from build123d import *

# Parameters (mm, degrees)
SKETCH1_R           = 1.5
BOSS_EXTRUDE3_DEPTH = 15
SKETCH3_R           = 1.5
CUT_EXTRUDE1_DEPTH  = 7.5
SKETCH5_W           = 13
SKETCH5_H           = 24
CUT_EXTRUDE2_DEPTH  = 10
SKETCH6_R           = 1
CUT_EXTRUDE3_DEPTH  = 10
SKETCH8_R           = 5.15
CUT_EXTRUDE4_DEPTH  = 15
SKETCH9_W           = 3
SKETCH9_H           = 13
CUT_EXTRUDE5_DEPTH  = 16
FILLET2_R           = 2
SKETCH10_W          = 6
SKETCH10_H          = 1.8
CUT_EXTRUDE6_DEPTH  = 16
SKETCH11_R          = 0.75
CUT_EXTRUDE7_DEPTH  = 10
SKETCH13_R          = 1.5
CUT_EXTRUDE8_DEPTH  = 16
SKETCH14_R          = 3
CUT_EXTRUDE9_DEPTH  = 5
SKETCH15_W          = 9
SKETCH15_H          = 15
SKETCH15_R          = 1.15
BOSS_EXTRUDE4_DEPTH = 2
SKETCH16_W          = 31.135337716
SKETCH16_H          = 16.721473769
CUT_EXTRUDE10_DEPTH = 16
CUT_EXTRUDE11_DEPTH = 20


with BuildPart() as part:
    # Sketch1 → Boss-Extrude3 (new body)
    with BuildSketch(Plane(origin=(0, 0, 0), x_dir=(1, 0, 0), z_dir=(0, 1, 0))):
        with BuildLine():
            Line((17, 40), (17, -19))
            Line((17, -19), (-17, -19))
            Line((-17, -19), (-17, 40))
            ThreePointArc((-17, 40), (-14.071067812, 47.071067812), (-7, 50))
            Line((-7, 50), (7, 50))
            ThreePointArc((7, 50), (14.071067812, 47.071067812), (17, 40))
        make_face()
        with Locations((-9, 0)):
            Circle(SKETCH1_R, mode=Mode.SUBTRACT)
        with Locations((9, 0)):
            Circle(SKETCH1_R, mode=Mode.SUBTRACT)
    extrude(amount=BOSS_EXTRUDE3_DEPTH)

    # Sketch3 → Cut-Extrude1 (cut)
    with BuildSketch(Plane(origin=(0, 15, 0), x_dir=(1, 0, 0), z_dir=(0, 1, 0))):
        with Locations((-11, 43)):
            Circle(SKETCH3_R)
        with Locations((11, 43)):
            Circle(SKETCH3_R)
        with BuildLine():
            Line((6, 48), (-6, 48))
            Line((-6, 48), (-6, 43))
            ThreePointArc((-6, 43), (-7.171572875, 40.171572875), (-10, 39))
            Line((-10, 39), (-15, 39))
            Line((-15, 39), (-15, 6))
            Line((-15, 6), (15, 6))
            Line((15, 6), (15, 39))
            Line((15, 39), (10, 39))
            ThreePointArc((10, 39), (7.171572875, 40.171572875), (6, 43))
            Line((6, 43), (6, 48))
        make_face()
    extrude(amount=-CUT_EXTRUDE1_DEPTH, mode=Mode.SUBTRACT)

    # Sketch5 → Cut-Extrude2 (cut)
    with BuildSketch(Plane(origin=(0, 7.5, 0), x_dir=(1, 0, 0), z_dir=(0, 1, 0))):
        with Locations((0, 27)):
            Rectangle(SKETCH5_W, SKETCH5_H)
    extrude(amount=-CUT_EXTRUDE2_DEPTH, mode=Mode.SUBTRACT)

    # Sketch6 → Cut-Extrude3 (cut)
    with BuildSketch(Plane(origin=(0, 7.5, 0), x_dir=(1, 0, 0), z_dir=(0, 1, 0))):
        with Locations((0, 41.1)):
            Circle(SKETCH6_R)
        with Locations((0, 12.9)):
            Circle(SKETCH6_R)
    extrude(amount=-CUT_EXTRUDE3_DEPTH, mode=Mode.SUBTRACT)

    # Sketch8 → Cut-Extrude4 (cut)
    with BuildSketch(Plane(origin=(0, 15, 0), x_dir=(1, 0, 0), z_dir=(0, 1, 0))):
        with Locations((-6, -12)):
            Circle(SKETCH8_R)
        with Locations((6, -12)):
            Circle(SKETCH8_R)
    extrude(amount=-CUT_EXTRUDE4_DEPTH, mode=Mode.SUBTRACT)

    # Sketch9 → Cut-Extrude5 (cut, through all)
    with BuildSketch(Plane(origin=(0, 15, 0), x_dir=(1, 0, 0), z_dir=(0, 1, 0))):
        with Locations((15.5, -12.5)):
            Rectangle(SKETCH9_W, SKETCH9_H)
        with Locations((-15.5, -12.5)):
            Rectangle(SKETCH9_W, SKETCH9_H)
    extrude(amount=-CUT_EXTRUDE5_DEPTH, mode=Mode.SUBTRACT)

    # Fillet2
    fillet2_edges = [part.edges().sort_by_distance(p)[0] for p in [
        (14, 7.5, 19),
        (-14, 7.5, 19),
    ]]
    fillet(fillet2_edges, radius=FILLET2_R)

    # Sketch10 → Cut-Extrude6 (cut, through all)
    with BuildSketch(Plane(origin=(0, 15, 0), x_dir=(1, 0, 0), z_dir=(0, 1, 0))):
        with Locations((0, -18.1)):
            Rectangle(SKETCH10_W, SKETCH10_H)
    extrude(amount=-CUT_EXTRUDE6_DEPTH, mode=Mode.SUBTRACT)

    # Sketch11 → Cut-Extrude7 (cut)
    with BuildSketch(Plane.XY.offset(17.2)):
        with Locations((0, 7.5)):
            Circle(SKETCH11_R)
    extrude(amount=-CUT_EXTRUDE7_DEPTH, mode=Mode.SUBTRACT)

    # Sketch13 → Cut-Extrude8 (cut, through all)
    with BuildSketch(Plane(origin=(0, 15, 0), x_dir=(1, 0, 0), z_dir=(0, 1, 0))):
        with Locations((11, 43)):
            Circle(SKETCH13_R)
        with Locations((-11, 43)):
            Circle(SKETCH13_R)
    extrude(amount=-CUT_EXTRUDE8_DEPTH, mode=Mode.SUBTRACT)

    # Sketch14 → Cut-Extrude9 (cut)
    with BuildSketch(Plane.XZ):
        with Locations((11, -43)):
            Circle(SKETCH14_R)
        with Locations((-11, -43)):
            Circle(SKETCH14_R)
    extrude(amount=-CUT_EXTRUDE9_DEPTH, mode=Mode.SUBTRACT)

    # Sketch15 → Boss-Extrude4 (add)
    with BuildSketch(Plane.XY.offset(19)):
        with Locations((7.5, 7.5)):
            Rectangle(SKETCH15_W, SKETCH15_H)
        with Locations((8, 12)):
            Circle(SKETCH15_R, mode=Mode.SUBTRACT)
    extrude(amount=BOSS_EXTRUDE4_DEPTH)

    # Sketch16 → Cut-Extrude10 (cut, through all)
    with BuildSketch(Plane(origin=(0, 15, 0), x_dir=(1, 0, 0), z_dir=(0, 1, 0))):
        with Locations((1.567668858, -14.360736885)):
            Rectangle(SKETCH16_W, SKETCH16_H)
    extrude(amount=-CUT_EXTRUDE10_DEPTH, mode=Mode.SUBTRACT)

    # Sketch19 → Cut-Extrude11 (cut)
    with BuildSketch(Plane.XY.offset(6)):
        with BuildLine():
            Line((3, 15), (13, 15))
            Line((13, 15), (13, 5))
            ThreePointArc((13, 5), (8, 2.022346613), (3, 5))
            Line((3, 5), (3, 15))
        make_face()
    extrude(amount=-CUT_EXTRUDE11_DEPTH, mode=Mode.SUBTRACT)


solid = part.part
Design review of the part built by this model. Coordinates are the model's own, in mm. A direction names the side the tool comes from. Give positions to 0.01 mm unless a question says otherwise; leave off trailing zeros. Order: outer loops, then holes, each group sorted by start corner. A loop starts at its lowest first (then second) coordinate and runs counter-clockwise, first axis right, second up.
1. Add section D-D, the plane y = 10.25. State the section outline as (x, z) points, then the cut area to 3 significant figures.
Solution:
outline: (-17, -40) arc R10 ccw to (-7, -50) - (7, -50) arc R10 ccw to (17, -40) - (17, 6) - (13, 6) - (13, -6) - (15, -6) - (15, -39) - (10, -39) arc R4 ccw to (6, -43) - (6, -48) - (-6, -48) - (-6, -43) arc R4 ccw to (-10, -39) - (-15, -39) - (-15, -6) - (3, -6) - (3, 6) - (-17, 6) - close; hole circle Ø3 at (-11, -43); hole circle Ø3 at (-9, 0); hole circle Ø3 at (11, -43)
area: 615 mm2
2. Add section A-A, the plane z = -37. State the section outline as (x, y) points.
Solution:
outline: (-17, 0) - (-6.5, 0) - (-6.5, 7.5) - (-15, 7.5) - (-15, 15) - (-17, 15) - close; (6.5, 0) - (17, 0) - (17, 15) - (15, 15) - (15, 7.5) - (6.5, 7.5) - close
3. Add section C-C, the plane y = 6. State the section outline as (x, z) points.
Solution:
outline: (-17, -40) arc R10 ccw to (-7, -50) - (7, -50) arc R10 ccw to (17, -40) - (17, 6) - (13, 6) - (13, -14) - (3, -14) - (3, 6) - (-17, 6) - close; hole circle Ø3 at (-11, -43); hole circle Ø3 at (-9, 0); hole (-6.5, -39) - (6.5, -39) - (6.5, -15) - (-6.5, -15) - close; hole circle Ø2 at (0, -41.1); hole circle Ø2 at (0, -12.9); hole circle Ø3 at (11, -43)
4. Add section B-B, the plane x = 0. State the section outline as (y, z) points, then the cut area to 3 significant figures.
Solution:
outline: (0, -50) - (15, -50) - (15, -48) - (7.5, -48) - (7.5, -42.1) - (0, -42.1) - close; (0, -40.1) - (7.5, -40.1) - (7.5, -39) - (0, -39) - close; (0, -15) - (7.5, -15) - (7.5, -13.9) - (0, -13.9) - close; (0, -11.9) - (7.5, -11.9) - (7.5, -6) - (15, -6) - (15, 6) - (0, 6) - close
area: 315 mm2
5. Mouldability with a two-part tool opening along X and no side actions: class faces 5 (the cylindrical face through (8.086, 2.023, -3.86)), 6 (the cylindrical face through (-13.21, 2.46, -40.97)), 7 (the cylindrical face through (-14.15, 7.4, -46.99)) as +X half, -X half, draft (parallel to the pull), parting line (faces both ways), or undercut.
Solution:
face 5: undercut
face 6: undercut
face 7: -X half
6. Tool access review of faces 1 (the cylindrical face through (11, 2, -40)), 2 (the flat face through (6.5, 4, -27)), 3 (the flat face through (-15, 11, -23)), 4 (the flat face through (3, 9, -2)): name each direction out of +Z, -Z, +X, -X, +Y, -Y from which nothing blocks a thin tool from reaching the whole face with its end or side.
Solution:
face 1: -Y
face 2: +Y, -Y
face 3: +Y
face 4: +Z, +Y
7. For pin 1 Ø1 at (x, y) = (12.5, 12.5) entering from -Z; pin 2 Ø4 at (x, y) = (-10.5, 11.5) entering from -Z; pin 3 Ø2 at (x, y) = (13.5, 11) entering from -Z, all flat-tipped, find the tip position at first contact; note any pin that passes through.
Solution:
pin 1: stops at z = -48.66
pin 2: stops at z = -49.89
pin 3: stops at z = -48.35
8. To check wall thickness, follow L1, parallel to X at y = 10.25, z = 0; L2, parallel to X at y = 10.5, z = 2; L3, parallel to X at y = 5, z = -22. State the ranges of each line that lie inside material, in increasing order.
Solution:
L1: x = -17 to -10.5, -7.5 to 3, 13 to 17
L2: x = -17 to 3, 13 to 17
L3: x = -17 to -6.5, 6.5 to 17
